Work out the finished part from the listing and answer in its coordinate system (mm). Give positions to 0.01 mm unless a question says otherwise; leave off trailing zeros. Write each loop counter-clockwise with the first axis right and the second up, starting at its lowest first coordinate (ties: lowest second). Pieces come first, ordered by that corner, then holes.
1) Straight lines are drawn through the part: probe 1 along Y at (x, z) = (-0.3, -193); probe 2 along Y at (x, z) = (-0.1, 171); probe 3 along Z at (x, y) = (-0.7, -144). For each, find the intervals that lie inside material, in ascending order.
2) Find section B-B (z = 169.5). Determine the outline of the cut face in (x, y).
3) Find section A-A (x = 0.25). Count the separate pieces of the cut face and the enclosed holes in it, plus the area to 3 significant figures.
4) Find section C-C (z = -208.5). Determine the outline of the cut face in (x, y), plus the area to 3 significant figures.
5) Given pin 1 Ø1.6 at (x, y) = (0, -139.5) entering from +Z; pin 2 Ø3 at (y, z) = (-142.9, -152) entering from +X; pin 3 Ø1.5 at (x, z) = (-0.5, 176.5) entering from -Y, each flat-ended and moving along its own axis, determine where each tip first touches the part or whether it passes through.
```python
from build123d import *

# Parameters (mm, degrees)
SKETCH1_W           = 498.348
SKETCH1_H           = 177.8
BOSS_EXTRUDE1_DEPTH = 1.5875
BOSS_EXTRUDE2_DEPTH = 3.175
SKETCH3_R           = 2.025
CUT_EXTRUDE1_DEPTH  = 307.121875894
LPATTERN1_COUNT     = 4
LPATTERN1_PITCH     = 76.2
CUT_EXTRUDE2_DEPTH  = 307.121875894
LPATTERN2_COUNT     = 2
LPATTERN2_PITCH     = 44.45
SKETCH5_R           = 2.025
CUT_EXTRUDE3_DEPTH  = 307.121875894
SKETCH8_R           = 2.025
CUT_EXTRUDE5_DEPTH  = 307.121875894
SKETCH9_R           = 2.025
CUT_EXTRUDE6_DEPTH  = 307.121875894
LPATTERN4_COUNT     = 2
LPATTERN4_PITCH     = 33.02


with BuildPart() as part:
    # Sketch1 → Boss-Extrude1 (new, symmetric)
    with BuildSketch(Plane(origin=(0, 0, 0), x_dir=(0, 0, -1), z_dir=(1, 0, 0))):
        Rectangle(SKETCH1_W, SKETCH1_H)
    extrude(amount=BOSS_EXTRUDE1_DEPTH, both=True)

    # Sketch2 → Boss-Extrude2 (add)
    with BuildSketch(Plane(origin=(1.5875, 0, 0), x_dir=(0, 0, -1), z_dir=(1, 0, 0))):
        Polygon((249.174, -95.25), (249.174, -88.9), (48.2854, -88.9), (48.2854, -177.8), (149.8854, -177.8), (185.674, -95.25), align=None)
    extrude(amount=-BOSS_EXTRUDE2_DEPTH)

    # Sketch3 → Cut-Extrude1 (cut, through all)
    with BuildSketch(Plane(origin=(1.5875, 0, 0), x_dir=(0, 0, -1), z_dir=(1, 0, 0))):
        with Locations((15.7854, -74.363480824)):
            Circle(SKETCH3_R)
    cut_extrude1 = extrude(amount=-CUT_EXTRUDE1_DEPTH, mode=Mode.SUBTRACT)

    # LPattern1: Cut-Extrude1 ×4
    with Locations(*[(0, 0, i * LPATTERN1_PITCH) for i in range(1, LPATTERN1_COUNT)]):
        add(cut_extrude1, mode=Mode.SUBTRACT)

    # Sketch4 → Cut-Extrude2 (cut, through all)
    with BuildSketch(Plane.ZY.offset(1.5875)):
        with BuildLine():
            ThreePointArc((-67.8504, -162.052), (-71.307291232, -160.620108768), (-69.8754, -164.077))
            Line((-69.8754, -164.077), (-69.8754, -162.052))
            Line((-69.8754, -162.052), (-67.8504, -162.052))
        make_face()
        with BuildLine():
            Line((-69.8754, -162.052), (-69.8754, -164.077))
            ThreePointArc((-69.8754, -164.077), (-68.443508768, -163.483891232), (-67.8504, -162.052))
            Line((-67.8504, -162.052), (-69.8754, -162.052))
        make_face()
    cut_extrude2 = extrude(amount=-CUT_EXTRUDE2_DEPTH, mode=Mode.SUBTRACT)

    # LPattern2: Cut-Extrude2 ×2
    with Locations(*[(0, 0, -i * LPATTERN2_PITCH) for i in range(1, LPATTERN2_COUNT)]):
        add(cut_extrude2, mode=Mode.SUBTRACT)

    # Sketch5 → Cut-Extrude3 (cut, through all)
    with BuildSketch(Plane.ZY.offset(1.5875)):
        with Locations((-152.00472504, -142.898934489)):
            Circle(SKETCH5_R)
    extrude(amount=-CUT_EXTRUDE3_DEPTH, mode=Mode.SUBTRACT)

    # Sketch8 → Cut-Extrude5 (cut, through all)
    with BuildSketch(Plane.ZY.offset(1.5875)):
        with Locations((-164.117120252, -110.224827622)):
            Circle(SKETCH8_R)
    extrude(amount=-CUT_EXTRUDE5_DEPTH, mode=Mode.SUBTRACT)

    # Sketch9 → Cut-Extrude6 (cut, through all)
    with BuildSketch(Plane.ZY.offset(1.5875)):
        with Locations((-201.170653386, -82.55)):
            Circle(SKETCH9_R)
    cut_extrude6 = extrude(amount=-CUT_EXTRUDE6_DEPTH, mode=Mode.SUBTRACT)

    # LPattern4: Cut-Extrude6 ×2
    with Locations(*[(0, 0, -i * LPATTERN4_PITCH) for i in range(1, LPATTERN4_COUNT)]):
        add(cut_extrude6, mode=Mode.SUBTRACT)


solid = part.part
```
Results:
1. probe 1: y = -95.25 to 88.9
1. probe 2: y = -88.9 to 88.9
1. probe 3: z = -164.54 to -153.7, -150.31 to -48.29
2. outline: (-1.59, -88.9) - (1.59, -88.9) - (1.59, 88.9) - (-1.59, 88.9) - close
3. separate pieces: 1
3. enclosed holes: 10
3. area: 99,600 mm2
4. outline: (-1.59, -95.25) - (1.59, -95.25) - (1.59, 88.9) - (-1.59, 88.9) - close
4. area: 585 mm2
5. pin 1: stops at z = -48.29
5. pin 2: passes through
5. pin 3: stops at y = -88.9
